Could you check a few things on this model? Use its own coordinates, in mm. A direction names the side the tool comes from. Coordinates: 2 decimals unless noted, no trailing zeros. Write each loop counter-clockwise with the first axis right and the second up, starting at its lowest first coordinate (ties: lowest second). Pieces come first, ordered by that corner, then holes. Notation, with made-up numbers: M 11.25,49.25 L 68.25,49.25 A15 ccw 68.25,67.25 Z; hole C 86,-19.5 d9. An arc over 180 degrees is marked long. Write item = value, one per line.
```python
from build123d import *

# Parameters (mm, degrees)
BOSS_EXTRUDE1_DEPTH = 30
CHAMFER1_SIZE       = 2
FILLET1_R           = 10
SKETCH2_W           = 10.333333333
SKETCH2_H           = 9
SKETCH2_W_2         = 10.333333334
CUT_EXTRUDE1_DEPTH  = 43.299527184
CUT_EXTRUDE2_DEPTH  = 3.2
SKETCH7_R           = 2.75
CUT_EXTRUDE3_DEPTH  = 2.8


with BuildPart() as part:
    # Sketch1 → Boss-Extrude1 (new, symmetric)
    with BuildSketch(Plane(origin=(0, 0, 0), x_dir=(0, 0, -1), z_dir=(1, 0, 0))):
        with BuildLine():
            Line((4.5, 0), (4.5, -12.5))
            Line((4.5, -12.5), (-24.5, -12.5))
            Line((-24.5, -12.5), (-24.5, -6.5))
            Line((-24.5, -6.5), (-4.5, -6.5))
            Line((-4.5, -6.5), (-4.5, 0))
            ThreePointArc((-4.5, 0), (0, 4.5), (4.5, 0))
        make_face()
    extrude(amount=BOSS_EXTRUDE1_DEPTH, both=True)

    # Chamfer1
    chamfer1_edges = [part.edges().sort_by_distance(p)[0] for p in [
        (0, -12.5, -4.5),
    ]]
    chamfer(chamfer1_edges, length=CHAMFER1_SIZE)

    # Fillet1
    fillet1_edges = [part.edges().sort_by_distance(p)[0] for p in [
        (-30, -9.5, 24.5),
        (30, -9.5, 24.5),
    ]]
    fillet(fillet1_edges, radius=FILLET1_R)

    # Sketch2 → Cut-Extrude1 (cut, through all)
    with BuildSketch(Plane.XZ.offset(12.5)):
        with Locations((-24.833333334, 0)):
            Rectangle(SKETCH2_W, SKETCH2_H)
        with Locations((-5, 0)):
            Rectangle(SKETCH2_W_2, SKETCH2_H)
        with Locations((14.833333334, 0)):
            Rectangle(SKETCH2_W, SKETCH2_H)
    extrude(amount=-CUT_EXTRUDE1_DEPTH, mode=Mode.SUBTRACT)

    # Sketch5 → CBORE for M3 Hex Socket Head Cap Screw1 (revolve, cut)
    with BuildSketch(Plane(origin=(30, 0, 0), x_dir=(0, 0, -1), z_dir=(0, 1, 0))):
        Polygon((0, 0), (0, 60), (1.7, 60), (1.7, 3.9), (3.25, 3.9), (3.25, 0.025), (3.275, 0), align=None)
    revolve(axis=Axis((36.35, 0, 0), (-1, 0, 0)), mode=Mode.SUBTRACT)

    # Sketch6 → Cut-Extrude2 (cut)
    with BuildSketch(Plane.XZ.offset(12.5)):
        Polygon((24.792007234, 14.5), (22.396003617, 18.65), (17.603996383, 18.65), (15.207992766, 14.5), (17.603996383, 10.35), (22.396003617, 10.35), align=None)
        Polygon((-15.207992766, 14.5), (-17.603996383, 18.65), (-22.396003617, 18.65), (-24.792007234, 14.5), (-22.396003617, 10.35), (-17.603996383, 10.35), align=None)
    extrude(amount=-CUT_EXTRUDE2_DEPTH, mode=Mode.SUBTRACT)

    # Sketch7 → Cut-Extrude3 (cut)
    with BuildSketch(Plane.XZ.offset(9.3)):
        with Locations(Location((-20, 14.5, 0), (0, 0, 270))):
            Circle(SKETCH7_R)
        with Locations(Location((20, 14.5, 0), (0, 0, 270))):
            Circle(SKETCH7_R)
    extrude(amount=-CUT_EXTRUDE3_DEPTH, mode=Mode.SUBTRACT)


solid = part.part
```
Item 1: For faces 1 (the face through (9.667, -4, 0)), 2 (the face through (-23.61, -10.92, 12.45)), 3 (the face through (-15, -3, 4.5)), 4 (the face through (25, -12, -3)), 5 (the face through (26.1, 1.4, 1.4)), which set-ups out of +Z, -Z, +X, -X, +Y, -Y let a thin tool reach every point of the face, with its end or its side?
Numbers:
face_1 = -Z, +Y, -Y
face_2 = -Y
face_3 = +Z, +X, -X, +Y
face_4 = -Z, +X, -X, -Y
face_5 = +X
Item 2: Imagine slicing it at A-A (z = 0). State how many separate pieces and enclosed holes the cut face has, and give its area (3 significant figures).
Numbers:
separate_pieces = 6
enclosed_holes = 0
area = 382 mm²
Item 3: If we mould it in two halves opening along Y, with no side actions, what happens to faces 6 (the face through (0, -12.5, 11)), 7 (the face through (-19.667, -4, 0)), 8 (the face through (5, 4.5, 0.1)), 9 (the face through (28.065, 1.978, 2.579))? For each: pulls with the +Y half, pulls with the -Y half, needs draft (parallel to the pull), parting line crosses it, or undercut.
Numbers:
face_6 = pulls with the -Y half
face_7 = needs draft
face_8 = pulls with the +Y half
face_9 = undercut
Item 4: I'm going to push flat-ended pins straight in: P1, Ø1.5, axis at x = -23.5, y = -10, coming from the -Z side; P2, Ø7, axis at y = -0.5, z = 1, coming from the -X side; P3, Ø6.5, axis at x = 19.5, z = 16.5, coming from the -Y side; P4, Ø7, axis at x = -20, z = 14.5, coming from the -Y side. Where does each tip first touch, or does it pass through?
Numbers:
P1 = 4.5
P2 = -19.67
P3 = -12.5
P4 = -9.3
Item 5: If I drill on line 1 along X through (y, z) = (-11.25, -1.25); line 2 along X through (y, z) = (-0.5, -2.5); line 3 along Y through (x, z) = (20.5, 0), over which ranges is the centre line in solid material (lowest first)?
Numbers:
line_1 = -19.67 to -10.17, 0.17 to 9.67, 20 to 30
line_2 = -19.67 to -10.17, 0.17 to 9.67, 20 to 26.1
line_3 = -12.5 to -1.7, 1.7 to 4.5
Item 6: Imagine slicing it at D-D (x = -6). Write out the boundary of the cut face in (y, z).
Numbers:
outline = M -12.5,4.5 L -6.5,4.5 L -6.5,24.5 L -12.5,24.5 Z
Item 7: Imagine slicing it at C-C (z = 16.5). Write out the boundary of the cut face in (x, y), and give its area (3 significant figures).
Numbers:
outline = M -29.8,-12.5 L -23.64,-12.5 L -23.64,-9.3 L -21.89,-9.3 L -21.89,-6.5 L -29.8,-6.5 Z; M -18.11,-9.3 L -16.36,-9.3 L -16.36,-12.5 L 16.36,-12.5 L 16.36,-9.3 L 18.11,-9.3 L 18.11,-6.5 L -18.11,-6.5 Z; M 21.89,-9.3 L 23.64,-9.3 L 23.64,-12.5 L 29.8,-12.5 L 29.8,-6.5 L 21.89,-6.5 Z
area = 290 mm²
Item 8: Imagine slicing it at B-B (y = -5.5). Write out the boundary of the cut face in (x, z), and give its area (3 significant figures).
Numbers:
outline = M -19.67,-4.5 L -10.17,-4.5 L -10.17,4.5 L -19.67,4.5 Z; M 0.17,-4.5 L 9.67,-4.5 L 9.67,4.5 L 0.17,4.5 Z; M 20,-4.5 L 30,-4.5 L 30,4.5 L 20,4.5 Z
area = 261 mm²
